Verification items for the finished model (mm, model axes). Face numbers are marked on the shaded views. A direction names the side the tool comes from. Give positions to 0.01 mm unless a question says otherwise; leave off trailing zeros. Order: outer loops, then holes, each group sorted by start corner. A loop starts at its lowest first (then second) coordinate and runs counter-clockwise, first axis right, second up.
(1) Sectioned sample at C-C on y = 63.5. Record the cut outline in (x, z), plus the area to 3 significant figures.
(2) Gauge pin test, flat ends, axial feed: pin 1 (4 mm diameter, centred on x = 0, y = 82, fed in from +Z); pin 2 (6 mm diameter, centred on x = 2, y = 54.5, fed in from -Z). Record the tip position at first contact, or that the pin passes through.
(3) Sectioned sample at A-A on z = 2.5. Record the cut outline in (x, y), plus the area to 3 significant figures.
(4) Sectioned sample at B-B on x = 0. Record the cut outline in (y, z).
(5) Access from +Z, -Z, +X, -X, +Y, -Y to the whole of each face (thin tool, end or side, straight path). Record for the marked faces 4 and 5.
(6) Mould release check, pull along Y, two halves, no side actions. Record for the marked faces 1, 2 and 3: pulls with the +Y half, pulls with the -Y half, needs draft (parallel to the pull), parting line crosses it, or undercut.
(7) Sectioned sample at D-D on y = 0. Record the cut outline in (x, z), plus the area to 3 significant figures.
(8) Scan lines: L1, parallel to Y at x = 0, z = 26.8; L2, parallel to X at y = 82, z = 7.5; L3, parallel to Y at x = 0, z = 11.5. Record each from-to range of solid material in increasing order.
```python
from build123d import *
from build123d.topology import SkipClean

# Parameters (mm, degrees)
SCHIZZO1_W                   = 10
SCHIZZO1_H                   = 10
SCHIZZO1_R                   = 2
ESTRUSIONE_ESTRUSIONE1_DEPTH = 25
SCHIZZO2_W                   = 10
SCHIZZO2_H                   = 92
SCHIZZO2_R                   = 1.75
SCHIZZO2_R_2                 = 2
ESTRUSIONE_ESTRUSIONE2_DEPTH = 5
ESTRUSIONE_ESTRUSIONE3_START = 25
SCHIZZO3_W                   = 10
SCHIZZO3_H                   = 10
SCHIZZO3_R                   = 1.75
ESTRUSIONE_ESTRUSIONE3_DEPTH = 25
SCHIZZO4_R                   = 4
TAGLIO_ESTRUSIONE1_DEPTH     = 5
RACCORDO1_R                  = 2


with BuildPart() as part:
    # Schizzo1 → Estrusione-Estrusione1 (new body)
    with BuildSketch(Plane.XY):
        Rectangle(SCHIZZO1_W, SCHIZZO1_H)
        Circle(SCHIZZO1_R, mode=Mode.SUBTRACT)
    extrude(amount=ESTRUSIONE_ESTRUSIONE1_DEPTH)

    # Schizzo2 → Estrusione-Estrusione2 (add)
    with BuildSketch(Plane.XY.offset(25)):
        with Locations((0, 41)):
            Rectangle(SCHIZZO2_W, SCHIZZO2_H)
        with Locations((0, 82)):
            Circle(SCHIZZO2_R, mode=Mode.SUBTRACT)
        Circle(SCHIZZO2_R_2, mode=Mode.SUBTRACT)
    extrude(amount=ESTRUSIONE_ESTRUSIONE2_DEPTH)

    # Schizzo3 → Estrusione-Estrusione3 (add)
    with SkipClean():  # the faces are left unmerged after this step: merging them gives an invalid solid
        with BuildSketch(Plane(origin=(0, 0, 25), x_dir=(-1, 0, 0), z_dir=(0, 0, -1)).offset(ESTRUSIONE_ESTRUSIONE3_START)):
            with Locations((0, 82)):
                Rectangle(SCHIZZO3_W, SCHIZZO3_H)
            with Locations((0, 82)):
                Circle(SCHIZZO3_R, mode=Mode.SUBTRACT)
        extrude(amount=-ESTRUSIONE_ESTRUSIONE3_DEPTH)

    # Schizzo4 → Taglio-Estrusione1 (cut)
    with BuildSketch(Plane.XY.offset(30)):
        Circle(SCHIZZO4_R)
        with Locations((0, 82)):
            Circle(SCHIZZO4_R)
    extrude(amount=-TAGLIO_ESTRUSIONE1_DEPTH, mode=Mode.SUBTRACT)

    # Raccordo1
    # the kernel refuses this fillet: 2 mm, written as the material it takes off along each edge
    with BuildSketch(Plane(origin=(-5, 92, 30), x_dir=(1, 0, 0), z_dir=(0, -1, 0)), Plane(origin=(5, -10, 30), x_dir=(-1, 0, 0), z_dir=(0, 1, 0))) as raccordo1_piece_1:
        with BuildLine():
            CenterArc((RACCORDO1_R, -RACCORDO1_R), RACCORDO1_R, 90, 90)
            Line((0, -RACCORDO1_R), (0, 0))
            Line((0, 0), (RACCORDO1_R, 0))
        make_face()
    extrude(amount=102, mode=Mode.SUBTRACT)
    with BuildSketch(Plane(origin=(-10, -5, 30), x_dir=(0, 1, 0), z_dir=(1, 0, 0)), Plane(origin=(10, 87, 30), x_dir=(0, -1, 0), z_dir=(-1, 0, 0))) as raccordo1_piece_2:
        with BuildLine():
            CenterArc((RACCORDO1_R, -RACCORDO1_R), RACCORDO1_R, 90, 90)
            Line((0, -RACCORDO1_R), (0, 0))
            Line((0, 0), (RACCORDO1_R, 0))
        make_face()
    extrude(amount=20, mode=Mode.SUBTRACT)
    with BuildSketch(Plane(origin=(0, 0, 30), x_dir=(1, 0, 0), z_dir=(0, -1, 0))) as raccordo1_piece_3:
        with BuildLine():
            CenterArc((4 + RACCORDO1_R, -RACCORDO1_R), RACCORDO1_R, 90, 90)
            Line((4, -RACCORDO1_R), (4, 0))
            Line((4, 0), (4 + RACCORDO1_R, 0))
        make_face()
    revolve(axis=Axis((0, 0, 30), (0, 0, 1)), mode=Mode.SUBTRACT)
    with BuildSketch(Plane(origin=(0, 82, 30), x_dir=(1, 0, 0), z_dir=(0, -1, 0))) as raccordo1_piece_4:
        with BuildLine():
            CenterArc((4 + RACCORDO1_R, -RACCORDO1_R), RACCORDO1_R, 90, 90)
            Line((4 + RACCORDO1_R, 0), (4, 0))
            Line((4, 0), (4, -RACCORDO1_R))
        make_face()
    revolve(axis=Axis((0, 82, 30), (0, 0, 1)), mode=Mode.SUBTRACT)


solid = part.part
```
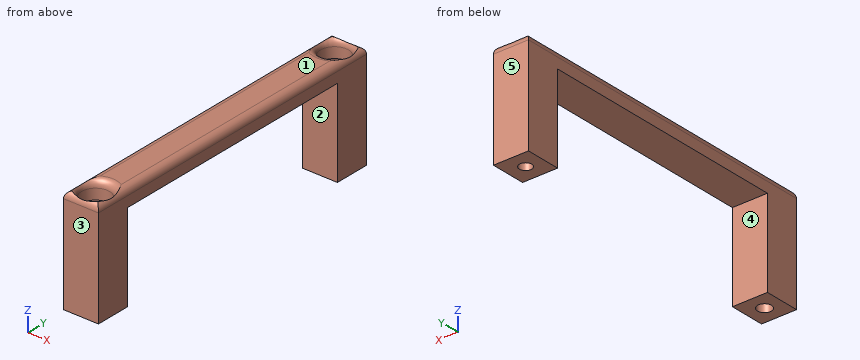
Ans:
1. outline: (-5, 25) - (5, 25) - (5, 28) arc R2 ccw to (3, 30) - (-3, 30) arc R2 ccw to (-5, 28) - close
1. area: 48.3 mm2
2. pin 1: stops at z = 25
2. pin 2: stops at z = 25
3. outline: (-5, -5) - (5, -5) - (5, 5) - (-5, 5) - close; (-5, 77) - (5, 77) - (5, 87) - (-5, 87) - close; hole circle Ø4 at (0, 0); hole circle Ø3.5 at (0, 82)
3. area: 178 mm2
4. outline: (-5, 0) - (-2, 0) - (-2, 25) - (-4, 25) - (-4, 28) arc R2 ccw to (-4.5, 29.32) arc R2 ccw to (-5, 28) - close; (2, 0) - (5, 0) - (5, 25) - (77, 25) - (77, 0) - (80.25, 0) - (80.25, 25) - (78, 25) - (78, 28) arc R2 ccw to (76, 30) - (6, 30) arc R2 ccw to (4, 28) - (4, 25) - (2, 25) - close; (83.75, 0) - (87, 0) - (87, 28) arc R2 ccw to (86.5, 29.32) arc R2 ccw to (86, 28) - (86, 25) - (83.75, 25) - close
5. face 4: -Z, +X, -X
5. face 5: +Z, -Z, +X, -X, +Y
6. face 1: needs draft
6. face 2: undercut
6. face 3: pulls with the -Y half
7. outline: (-5, 0) - (-2, 0) - (-2, 25) - (-4, 25) - (-4, 28) arc R2 ccw to (-4.5, 29.32) arc R2 ccw to (-5, 28) - close; (2, 0) - (5, 0) - (5, 28) arc R2 ccw to (4.5, 29.32) arc R2 ccw to (4, 28) - (4, 25) - (2, 25) - close
7. area: 158 mm2
8. L1: y = -5 to -4, 4 to 78, 86 to 87
8. L2: x = -5 to -1.75, 1.75 to 5
8. L3: y = -5 to -2, 2 to 5, 77 to 80.25, 83.75 to 87
